Can you work these out from the model? Positions are in its coordinate system, mm. Face numbers are marked on the shaded views. Round coordinates to 2 decimals unless told otherwise and drop trailing zeros. Loops run counter-clockwise (first coordinate to the right, second up) from the corner with the lowest first, then second, coordinate; pieces in that order, holes last. Notation, with made-up numbers: M -30,-22 L 21,-22 A15 ccw 21,6 Z; hole C -10.75,-11.5 d3. An arc over 180 degrees is marked long. Use a Markdown table: item, result. Add a question column.
```python
from build123d import *

# Parameters (mm, degrees)
F1_DEPTH = 34.925
F2_SIZE  = 22.22499
F3_SIZE  = 22.22499
F5_D     = 6.35
F6_D     = 6.35


# Not quite as in the source:
# - a fillet or chamfer is up to 0.001 mm smaller than in the source, because OpenCascade refuses the exact size


with BuildPart() as f1:
    # F0 (on Top) → F1 (new body, symmetric)
    with BuildSketch(Plane.XY):
        Polygon((-46.0238126205, -30.3083644086), (-30.3083644086, -46.0238126205), (46.0238126205, 30.3083644086), (30.3083644086, 46.0238126205), align=None)
    extrude(amount=F1_DEPTH, both=True)

    # F2 (size 22.225 in the source; OpenCascade refuses exactly that, so slightly less here)
    f2_edges = [f1.edges().sort_by_distance(p)[0] for p in [
        (46.023813, 30.308364, 0),
    ]]
    chamfer(f2_edges, length=F2_SIZE)

    # F3 (size 22.225 in the source; OpenCascade refuses exactly that, so slightly less here)
    f3_edges = [f1.edges().sort_by_distance(p)[0] for p in [
        (-30.308364, -46.023813, 0),
    ]]
    chamfer(f3_edges, length=F3_SIZE)

    # F5 (through all)
    with Locations(Plane(origin=(7.8577241059, -7.8577241059, 0), x_dir=(0.7071067812, 0.7071067812, 0), z_dir=(0.7071067812, -0.7071067812, 0))):
        with Locations((0, 19.05)):
            Hole(F5_D / 2)

    # F6 (through all)
    with Locations(Plane(origin=(7.8577241059, -7.8577241059, 0), x_dir=(0.7071067812, 0.7071067812, 0), z_dir=(0.7071067812, -0.7071067812, 0))):
        with Locations((0, -12.7)):
            Hole(F6_D / 2)


solid = f1.part
```
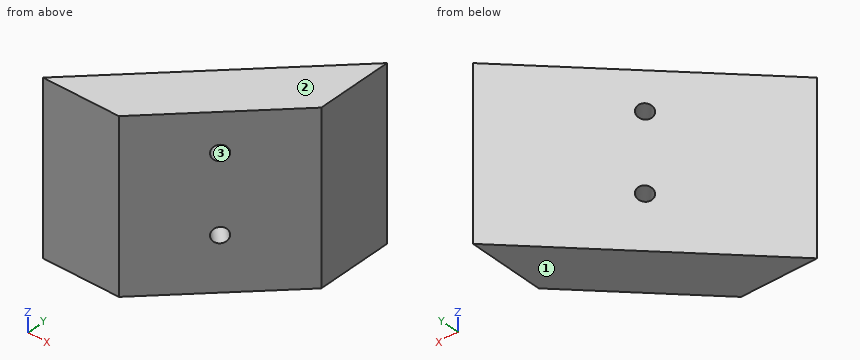
(1) Thinking about a two-plate mould opening in Z: for the marked faces 1, 2 and 3, which applies, released by +Z, released by -Z, zero draft, split by the parting line, or undercut?
(2) I'm going to push flat-ended pins straight in: pin 1 (1.5 mm diameter, centred on x = 22.5, z = 2.5, fed in from -Y); pin 2 (8 mm diameter, centred on y = 13.5, z = -27, fed in from -X); pin 3 (10 mm diameter, centred on x = -28, z = 6, fed in from +Y); pin 4 (10 mm diameter, centred on x = -9.5, y = 14.5, fed in from -Z). Where does each tip first touch, or does it pass through?
(3) If I drill on probe 1 along Z at (x, y) = (4, -4.5) (3 decimals); probe 2 along Y at (x, z) = (3.5, 18.5); probe 3 along Y at (x, z) = (4, 11.5), over which ranges is the centre line in solid material (lowest first)? Write a range as [from, to].
(4) Suppose I cut it at D-D on y = 4. Count the separate pieces of the cut face and the enclosed holes in it, and give its area (3 significant figures).
(5) Suppose I cut it at B-B on y = -25. List the corners of the cut face in (x, z) for me (3 decimals).
(6) Suppose I cut it at C-C on x = 14. List the corners of the cut face in (y, z) for me (3 decimals).
Results below:
| question | item | result |
|---|---|---|
| 1 | face 1 | released by -Z |
| 1 | face 2 | released by +Z |
| 1 | face 3 | undercut |
| 2 | pin 1 | stops at y = 6.03 |
| 2 | pin 2 | stops at x = -6.22 |
| 2 | pin 3 | stops at y = -7.28 |
| 2 | pin 4 | passes through |
| 3 | probe 1 | z = [-34.925, -15.855], [-9.545, 15.895], [22.205, 34.925] |
| 3 | probe 2 | y = [-12.22, -7.92], [0.92, 19.22] |
| 3 | probe 3 | y = [-11.72, 19.72] |
| 4 | separate pieces | 1 |
| 4 | enclosed holes | 2 |
| 4 | area | 2,110 mm² |
| 5 | outline | M -40.715,-34.925 L -9.285,-34.925 L -9.285,34.925 L -40.715,34.925 Z |
| 6 | outline | M -1.715,-34.925 L 29.715,-34.925 L 29.715,34.925 L -1.715,34.925 Z |
